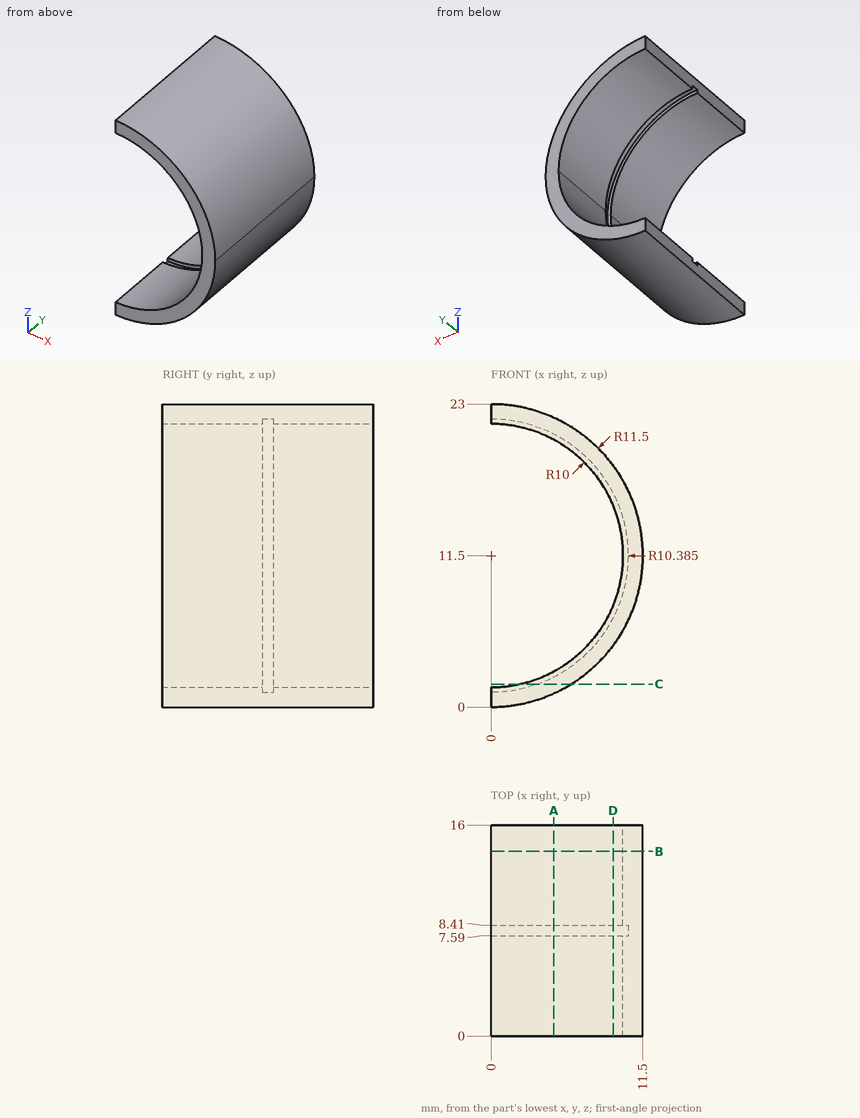
The drawing under review shows one solid part. Ordinate dimensions are in mm from its lowest x, y, z. Give positions to 0.01 mm unless a question says otherwise; leave off trailing zeros. Order: outer loops, then holes, each group sorted by start corner. A loop starts at its lowest first (then second) coordinate and runs counter-clockwise, first axis right, second up. Notation, with made-up numbers: (3, 52.25) -> (56, 52.25) arc R21 cw to (56, 77.25) -> close; hole circle Ø8 at (89, 86). An arc over 180 degrees is marked (long way). Write item = value, one per line. Start each with the question number.
(1) We need section B-B on y = 14. Write out the cut boundary in (x, z), plus the area to 3 significant figures.
(2) We need section A-A on x = 4.75. Write out the cut boundary in (y, z) (3 decimals).
(3) We need section C-C on z = 1.75. Write out the cut boundary in (x, y).
(4) For pin 1 (5 mm diameter, centred on x = 7, y = 3, fed in from -Z); pin 2 (1.5 mm diameter, centred on y = 11.5, z = 10.5, fed in from +X); pin 3 (1 mm diameter, centred on x = 9.5, z = 6.5, fed in from -Y); pin 4 (6 mm diameter, centred on x = 3, z = 5.5, fed in from +Y), all flat-tipped, find the tip position at first contact; note any pin that passes through.
(5) We need section D-D on x = 9.25. Write out the cut boundary in (y, z).
(6) To check wall thickness, follow line 1 along Y through (x, z) = (10.25, 12.75); line 2 along X through (y, z) = (7.25, 11.25); line 3 along Z through (x, y) = (9, 3). State the ranges of each line that lie inside material, in increasing order.
Numbers:
q1.outline = (0, 0) arc R11.5 ccw to (0, 23) -> (0, 21.5) arc R10 cw to (0, 1.5) -> close
q1.area = 50.7 mm^2
q2.outline = (0, 1.027) -> (16, 1.027) -> (16, 2.7) -> (8.41, 2.7) -> (8.41, 2.265) -> (7.59, 2.265) -> (7.59, 2.7) -> (0, 2.7) -> close; (0, 20.3) -> (7.59, 20.3) -> (7.59, 20.735) -> (8.41, 20.735) -> (8.41, 20.3) -> (16, 20.3) -> (16, 21.973) -> (0, 21.973) -> close
q3.outline = (2.22, 0) -> (6.1, 0) -> (6.1, 16) -> (2.22, 16) -> (2.22, 8.41) -> (3.58, 8.41) -> (3.58, 7.59) -> (2.22, 7.59) -> close
q4.pin_1 = 0.92
q4.pin_2 = 11.5
q4.pin_3 = 0
q4.pin_4 = through
q5.outline = (0, 4.67) -> (16, 4.67) -> (16, 7.7) -> (8.41, 7.7) -> (8.41, 6.78) -> (7.59, 6.78) -> (7.59, 7.7) -> (0, 7.7) -> close; (0, 15.3) -> (7.59, 15.3) -> (7.59, 16.22) -> (8.41, 16.22) -> (8.41, 15.3) -> (16, 15.3) -> (16, 18.33) -> (0, 18.33) -> close
q6.line_1 = 0 to 7.59, 8.41 to 16
q6.line_2 = 10 to 11.5
q6.line_3 = 4.34 to 7.14, 15.86 to 18.66
